```python
from build123d import *

# Parameters (mm, degrees)
F1_DEPTH = 10.16
F3_DEPTH = 12.7


with BuildPart() as f1:
    # F0 (on Front) → F1 (new body)
    with BuildSketch(Plane.XZ):
        Polygon((-43.755643, 90.828305), (-46.877941, 88.841388), (-48.722932, 86.428699), (-49.858313, 81.603329), (-52.271002, 77.771422), (-55.109454, 72.094509), (-59.367137, 66.985293), (-65.044043, 60.598771), (-72.424024, 54.354175), (-77.249394, 47.683807), (-80.22977, 44.561509), (-83.352068, 38.600758), (-86.332443, 32.214235), (-92.009354, 29.517705), (-97.686262, 30.795009), (-103.363165, 34.484999), (-104.49855, 37.465376), (-107.337004, 33.917309), (-107.337004, 29.659627), (-104.072782, 26.963097), (-100.240867, 24.834256), (-94.56396, 23.698875), (-88.603207, 23.698875), (-83.352068, 23.698875), (-80.22977, 26.963097), (-78.526698, 23.698875), (-70.153258, 23.698875), (-63.482894, 23.698875), (-61.495977, 25.543871), (-63.482894, 27.683625), (-59.367137, 26.963097), (-59.367137, 29.659627), (-61.495977, 31.504622), (-61.495977, 33.917309), (-55.109454, 36.329995), (-55.109454, 29.659627), (-52.271002, 25.543871), (-49.858313, 22.421573), (-45.458715, 22.421573), (-42.904107, 23.698875), (-43.826604, 25.543871), (-48.722932, 26.963097), (-41.342954, 26.963097), (-40.349492, 27.683625), (-45.458715, 31.220777), (-45.458715, 36.329995), (-45.458715, 43.284205), (-39.923728, 48.819191), (-35.382203, 53.502639), (-35.382203, 58.611854), (-35.382203, 64.146841), (-36.659504, 72.094509), (-36.659504, 74.932962), (-33.25336, 76.210269), (-29.421452, 76.210269), (-27.576454, 78.05526), (-28.711836, 79.616412), (-32.117979, 81.603329), (-28.002219, 81.603329), (-26.157228, 85.293318), (-26.157228, 86.428699), (-31.692215, 87.56408), (-35.382203, 87.56408), (-37.794885, 90.828305), align=None)
    extrude(amount=F1_DEPTH)

    # F2 (on face) → F3 (join)
    with BuildSketch(Plane.XZ.offset(10.16)):
        Polygon((-52.004732, 54.195438), (-60.263611, 54.195438), (-60.020704, 48.608549), (-52.004732, 48.608549), align=None)
    extrude(amount=F3_DEPTH)


solid = f1.part
```
Geometry check sheet. Reference: the model listing, model coordinates, mm. A direction names the side the tool comes from. Give positions to 0.01 mm unless a question says otherwise; leave off trailing zeros. Order: outer loops, then holes, each group sorted by start corner. A loop starts at its lowest first (then second) coordinate and runs counter-clockwise, first axis right, second up.
1. Section check B-B, the plane z = 83.5. Enter the section's corners in (x, y).
2. Gauge pin test, flat ends, axial feed: pin 1 Ø2 at (y, z) = (-7, 28) entering from +X; pin 2 Ø1.1 at (x, y) = (-33.5, -5.5) entering from +Z; pin 3 Ø4 at (y, z) = (-3, 69.5) entering from +X. Record the tip position at first contact, or that the pin passes through.
3. Release check for a two-part mould opening along X. For faces 6 (the face through (-51.05, -5.01, 79.71)), 7 (the face through (-79.39, -5.01, 25.35)), 8 (the face through (-58, 0, 50)), 9 (the face through (-100.48, -5.01, 32.61)) record: pulls with the +X half, pulls with the -X half, needs draft (parallel to the pull), parting line crosses it, or undercut.
4. Access from +Z, -Z, +X, -X, +Y, -Y to the whole of each face (thin tool, end or side, straight path). Record for faces 1 (the face through (-103.92, -5.01, 35.95)), 2 (the face through (-43.36, -5.01, 24.61)), 3 (the face through (-58.347, -5.009, 35.107)), 4 (the face through (-35.382, -5, 59)), 5 (the face through (-52.005, -16, 51)).
5. Thickness scan on L1, parallel to Y at x = -69.5, z = 27.5; L2, parallel to Z at x = -58, y = -10.25; L3, parallel to X at y = -2.25, z = 64. Record the ranges inside material, lowest first.
6. Section check A-A, the plane y = -15. Enter the section's corners in (x, z).
Values follow:
1. outline: (-49.41, -10.16) - (-27.05, -10.16) - (-27.05, 0) - (-49.41, 0) - close
2. pin 1: stops at x = -40.35
2. pin 2: stops at z = 87.56
2. pin 3: stops at x = -35.92
3. face 6: pulls with the -X half
3. face 7: undercut
3. face 8: needs draft
3. face 9: undercut
4. face 1: +Z, +Y, -Y
4. face 2: +X, +Y, -Y
4. face 3: +Y, -Y
4. face 4: -Z, +X, +Y, -Y
4. face 5: +Z, -Z, +X, -Y
5. L1: y = -10.16 to 0
5. L2: z = 48.61 to 54.2
5. L3: x = -62.02 to -35.38
6. outline: (-60.26, 54.2) - (-60.02, 48.61) - (-52, 48.61) - (-52, 54.2) - close
